Here's how the part is built. I have some questions about the finished solid (model axes, mm). A direction names the side the tool comes from. Give positions to 0.01 mm unless a question says otherwise; leave off trailing zeros. Order: outer loops, then holes, each group sorted by start corner. A loop starts at its lowest first (then second) coordinate and runs counter-clockwise, first axis right, second up.
Autodesk Fusion 360 part; units mm, degrees
sketch "Sketch1" plane through (0, 0, 0) normal (0, 0, 1) x (1, 0, 0)
  line L0 (15.25, -12.5) -> (-15.25, -12.5)
  line L1 (-15.25, -12.5) -> (-15.25, 12.5)
  line L2 (-15.25, 12.5) -> (15.25, 12.5)
  line L3 (15.25, 12.5) -> (15.25, -12.5)
  line L4 (15.25, -12.5) -> (-15.25, 12.5) construction
  line L5 (-15.25, -12.5) -> (15.25, 12.5) construction
  dimension "d1" = 30.5
  dimension "d2" = 25
extrude "Extrude1" add sketch "Sketch1" along normal blind 1
sketch "Sketch2" plane through (0, 12.5, 0) normal (0, 1, 0) x (-1, 0, 0)
  line L0 (-15.25, 0) -> (15.25, 0)
  line L1 (15.25, 0) -> (15.25, 1)
  line L2 (15.25, 1) -> (-15.25, 1)
  line L3 (-15.25, 1) -> (-15.25, 0)
  line L4 (15.25, 1) -> (-15.25, 1)
  line L5 (-15.25, 1) -> (-15.25, -45)
  line L6 (-15.25, -45) -> (15.25, -45)
  line L7 (15.25, -45) -> (15.25, 1)
  dimension "d5" = 46
  dimension "d6" = 30.5
extrude "Extrude2" add sketch "Sketch2" along normal blind 1
sketch "Sketch3" plane through (0, 0, 1) normal (0, 0, 1) x (1, 0, 0)
  line L0 (-15.25, 13.5) -> (-15.25, -12.5)
  line L1 (-15.25, -12.5) -> (15.25, -12.5)
  line L2 (15.25, -12.5) -> (15.25, 13.5)
  line L3 (15.25, 13.5) -> (-15.25, 13.5)
  line L4 (0, -12.5) -> (0, -5.95)
  circle A0 centre (0, -5.95) radius 3.75
  dimension "d9" = 6.55
  dimension "d10" = 7.5
extrude "Extrude3" cut sketch "Sketch3" against normal blind 46 contours A0
sketch "Sketch4" plane through (0, 13.5, 0) normal (0, 1, 0) x (-1, 0, 0)
  line L0 (15.25, -45) -> (15.25, 1)
  line L1 (15.25, 1) -> (-15.25, 1)
  line L2 (-15.25, 1) -> (-15.25, -45)
  line L3 (-15.25, -45) -> (15.25, -45)
  line L4 (0, 1) -> (0, -24.5)
  circle A0 centre (0, -24.5) radius 3.625
  dimension "d13" = 25.5
  dimension "d14" = 7.25
extrude "Extrude4" cut sketch "Sketch4" against normal blind 20 contours A0
equation "d9 = 2.8 mm + 3.75 mm"
Q1. If we section it at C-C on z = -24.5: List the corners of the cut face in (x, y) for me (3 decimals), plus the area to 4 significant figures.
Filled sheet:
outline: (-15.25, 12.5) - (-3.625, 12.5) - (-3.625, 13.5) - (-15.25, 13.5) - close; (3.625, 12.5) - (15.25, 12.5) - (15.25, 13.5) - (3.625, 13.5) - close
area: 23.25 mm2
Q2. If we section it at D-D on x = 13: List the corners of the cut face in (y, z) for me, plus the area to 3 significant figures.
Filled sheet:
outline: (-12.5, 0) - (12.5, 0) - (12.5, -45) - (13.5, -45) - (13.5, 1) - (-12.5, 1) - close
area: 71.0 mm2
Q3. Thinking about a two-plate mould opening in X: for faces 3 (the face through (-15.25, 13, -12)), 4 (the face through (-1.7, 13, -27.7)), 5 (the face through (15.25, 13, -12)), 6 (the face through (-3, 13.5, -22)), which applies, released by +X, released by -X, zero draft, split by the parting line, or undercut?
Filled sheet:
face 3: released by -X
face 4: undercut
face 5: released by +X
face 6: zero draft
Q4. I'm going to push flat-ended pins straight in: P1, Ø10, axis at y = 5, z = -6, coming from the -X side; P2, Ø5, axis at x = -5, z = -8.5, coming from the -Y side; P3, Ø8.5, axis at x = 0, y = -5.95, coming from the -Z side. Where does each tip first touch, or does it pass through?
Filled sheet:
P1: passes through
P2: stops at y = 12.5
P3: stops at z = 0
Q5. If we section it at A-A on y = -5.95: List the corners of the cut face in (x, z) for me, plus the area to 3 significant figures.
Filled sheet:
outline: (-15.25, 0) - (-3.75, 0) - (-3.75, 1) - (-15.25, 1) - close; (3.75, 0) - (15.25, 0) - (15.25, 1) - (3.75, 1) - close
area: 23.0 mm2
Q6. If we section it at B-B on x = 0: List the corners of the cut face in (y, z) for me (3 decimals).
Filled sheet:
outline: (-12.5, 0) - (-9.7, 0) - (-9.7, 1) - (-12.5, 1) - close; (-2.2, 0) - (12.5, 0) - (12.5, -20.875) - (13.5, -20.875) - (13.5, 1) - (-2.2, 1) - close; (12.5, -45) - (13.5, -45) - (13.5, -28.125) - (12.5, -28.125) - close
Q7. For faces 1 (the face through (0, 0, 0)), 2 (the face through (0, 1, 1)), which set-ups out of +Z, -Z, +X, -X, +Y, -Y let a thin tool reach every point of the face, with its end or its side?
Filled sheet:
face 1: -Z, +X, -X, -Y
face 2: +Z, +X, -X, +Y, -Y
Q8. I need wall thicknesses on L1, parallel to Y at x = 0, z = 0.55; L2, parallel to Z at x = 0, y = 12.7 (3 decimals); L3, parallel to X at y = -5.95, z = 0.3. Which ranges of each line are inside material? Lowest first, please.
Filled sheet:
L1: y = -12.5 to -9.7, -2.2 to 13.5
L2: z = -45 to -28.125, -20.875 to 1
L3: x = -15.25 to -3.75, 3.75 to 15.25
